Input: part model. Units: mm. Frame: model coordinates. Face numbers are marked on the shaded views. A direction names the side the tool comes from. Coordinates: 2 decimals unless noted, no trailing zeros. Order: outer loops, then holes, each group sorted by start corner. A loop starts at its lowest first (then second) coordinate and runs counter-clockwise, first axis right, second up. Notation, with made-up numbers: M -15.5,45 L 17.5,45 A25 ccw 17.5,63 Z; hole C 28.25,29 d7. An arc over 180 degrees is marked long. One line per item, written item: value.
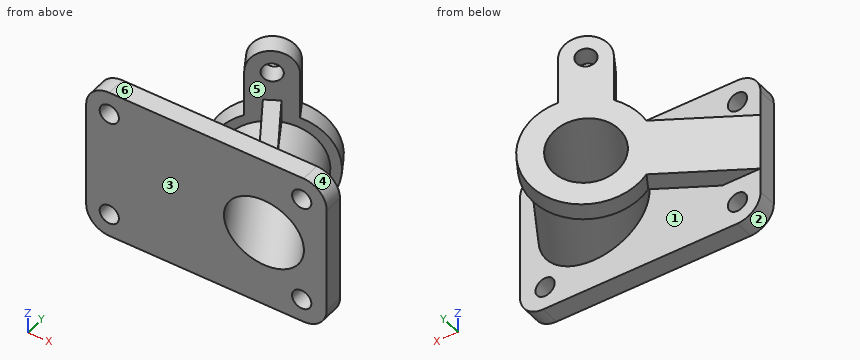
```python
from build123d import *

# Parameters (mm, degrees)
SKETCH_1_R          = 5
EXTRUDE_1_DEPTH     = 10
SKETCH_3_R          = 5
SKETCH_3_R_2        = 18
EXTRUDE_3_DEPTH     = 10
EXTRUDE_4_REACH     = 73.16
SKETCH_4_R          = 25
SKETCH_5_R          = 18
CUT_EXTRUDE_1_DEPTH = 72.160254038
EXTRUDE_6_DEPTH     = 4


with BuildPart() as part:
    # 草图1 → 凸台-拉伸1 (new body)
    with BuildSketch(Plane(origin=(0, 0, 0), x_dir=(1, 0, 0), z_dir=(0, 1, 0))):
        with BuildLine():
            Line((-69.708508874, 31.297621281), (31.291491126, 31.297621281))
            ThreePointArc((31.291491126, 31.297621281), (39.7767725, 27.782902656), (43.291491126, 19.297621281))
            Line((43.291491126, 19.297621281), (43.291491126, -36.702378719))
            ThreePointArc((43.291491126, -36.702378719), (39.7767725, -45.187660093), (31.291491126, -48.702378719))
            Line((31.291491126, -48.702378719), (-69.708508874, -48.702378719))
            ThreePointArc((-69.708508874, -48.702378719), (-78.193790248, -45.187660093), (-81.708508874, -36.702378719))
            Line((-81.708508874, -36.702378719), (-81.708508874, 19.297621281))
            ThreePointArc((-81.708508874, 19.297621281), (-78.193790248, 27.782902656), (-69.708508874, 31.297621281))
        make_face()
        with Locations((-69.708508874, -36.702378719)):
            Circle(SKETCH_1_R, mode=Mode.SUBTRACT)
        with Locations((30.291491126, -36.702378719)):
            Circle(SKETCH_1_R, mode=Mode.SUBTRACT)
        with Locations((30.291491126, 19.297621281)):
            Circle(SKETCH_1_R, mode=Mode.SUBTRACT)
        with Locations((-69.708508874, 19.297621281)):
            Circle(SKETCH_1_R, mode=Mode.SUBTRACT)
    extrude(amount=EXTRUDE_1_DEPTH)

    # 草图3 → 凸台-拉伸3 (add)
    with BuildSketch(Plane(origin=(-24.757254237, 42.880822195, 0), x_dir=(0, 0, 1), z_dir=(-0.5, 0.866025404, 0))):
        with BuildLine():
            Line((-6.297621281, -65.76164439), (-6.297621281, -16.742406504))
            ThreePointArc((-6.297621281, -16.742406504), (-11.289336226, 31.606443002), (36.197832888, 21.23835561))
            Line((36.197832888, 21.23835561), (60.702378719, 21.23835561))
            ThreePointArc((60.702378719, 21.23835561), (72.702378719, 9.23835561), (60.702378719, -2.76164439))
            Line((60.702378719, -2.76164439), (36.197832888, -2.76164439))
            ThreePointArc((36.197832888, -2.76164439), (31.070466111, -10.753359335), (23.702378719, -16.742406504))
            Line((23.702378719, -16.742406504), (23.702378719, -65.76164439))
            Line((23.702378719, -65.76164439), (-6.297621281, -65.76164439))
        make_face()
        with Locations((60.702378719, 9.23835561)):
            Circle(SKETCH_3_R, mode=Mode.SUBTRACT)
        with Locations((8.702378719, 9.23835561)):
            Circle(SKETCH_3_R_2, mode=Mode.SUBTRACT)
    extrude(amount=-EXTRUDE_3_DEPTH)

    # 草图4 → 凸台-拉伸4 (add, up to next)
    with BuildSketch(Plane(origin=(-24.757254237, 42.880822195, 0), x_dir=(0, 0, 1), z_dir=(-0.5, 0.866025404, 0)), mode=Mode.PRIVATE) as extrude_4_sk1:
        with Locations((8.702378719, 9.23835561)):
            Circle(SKETCH_4_R)
    extrude_4_tool1 = extrude(extrude_4_sk1.sketch, amount=-EXTRUDE_4_REACH, mode=Mode.PRIVATE) - part.part
    add(extrude_4_tool1.solids().sort_by_distance((-16.756604, 47.5, 8.702379))[0])

    # 草图5 → 切除-拉伸1 (cut, through all)
    with BuildSketch(Plane(origin=(-24.757254237, 42.880822195, 0), x_dir=(0.866025404, 0.5, 0), z_dir=(-0.5, 0.866025404, 0))):
        with Locations((9.23835561, -8.702378719)):
            Circle(SKETCH_5_R)
    extrude(amount=-CUT_EXTRUDE_1_DEPTH, mode=Mode.SUBTRACT)

    # 草图7 → 凸台-拉伸6 (add, symmetric)
    with BuildSketch(Plane(origin=(8.000650647, 4.619177805, 0), x_dir=(0, 0, 1), z_dir=(-0.866025404, -0.5, 0))):
        Polygon((45.297720901, 39.514508475), (30.011923646, 39.514508475), (30.472342637, 13.83620008), align=None)
    extrude(amount=EXTRUDE_6_DEPTH, both=True)


solid = part.part
```
(1) Access query for the marked faces 4, 5 and 6. Directions: +Z, -Z, +X, -X, +Y, -Y. A direction counts if a zero-diameter tool reaches every point of the face in a straight line with its end or side. Return the directions, or none.
Data:
face 4: +Z, +X, +Y, -Y
face 5: none
face 6: +Z, +X, -X, -Y
(2) First-contact query: pin 1 (8 mm diameter, centred on y = 16.5, z = -11, fed in from +X) (3 decimals); pin 2 (10 mm diameter, centred on x = 7.5, y = 56, fed in from +Z); pin 3 (1 mm diameter, centred on x = 27.5, z = 16, fed in from -Y); pin 4 (13 mm diameter, centred on x = 30.29, z = 36.7, fed in from -Y). Flat tips, straight axial feed; report the tip coordinate or a pass-through.
Data:
pin 1: stops at x = 24.245
pin 2: stops at z = 30.83
pin 3: stops at y = 2.78
pin 4: stops at y = 0
(3) Draft query along X for the marked faces 1, 2 and 3. Return one class per face: released by +X, released by -X, zero draft, split by the parting line, or undercut.
Data:
face 1: undercut
face 2: released by -X
face 3: zero draft
(4) Cut plane A-A on z = 16. Output: boundary loops of the cut face in (x, y).
Data:
outline: M -81.71,0 L -8.33,0 L -31.01,39.27 L -81.71,10 Z; M -2.51,55.73 L 29.67,0 L 43.29,0 L 43.29,10 L 32.5,10 L 8.95,50.8 L 13.44,53.39 L 8.44,62.05 Z; hole M -61.71,10 L -22.72,10 L -32.46,26.88 Z
(5) Cut plane C-C on x = -45. Output: boundary loops of the cut face in (y, z).
Data:
outline: M 0,-31.3 L 10,-31.3 L 10,48.7 L 0,48.7 Z; M 19.65,-6.3 L 31.19,-6.3 L 31.19,23.7 L 19.65,23.7 Z
(6) Cut plane B-B on x = -67. Output: boundary loops of the cut face in (y, z).
Data:
outline: M 0,-31.3 L 10,-31.3 L 10,-23.5 L 0,-23.5 Z; M 0,-15.09 L 10,-15.09 L 10,-6.3 L 18.49,-6.3 L 18.49,23.7 L 10,23.7 L 10,32.5 L 0,32.5 Z; M 0,40.91 L 10,40.91 L 10,48.7 L 0,48.7 Z
(7) Ray query, line 1 (Z direction, x = -13, y = 46); line 2 (Z direction, x = 8, y = 4); line 3 (X direction, y = 27, z = 0). Return the intervals inside material, ascending. Write a range as from..to.
Data:
line 1: z = -21.19..-9.12, 26.53..56.37, 65.03..72.44
line 2: z = -31.3..-9.29, 26.7..48.7
line 3: x = -52.26..-32.26, -31.98..-23.12, 13.27..22.14
(8) Cut plane D-D on z = 1.5. Output: boundary loops of the cut face in (x, y), plus the area to 3 significant figures.
Data:
outline: M -81.71,0 L -8.38,0 L -31.04,39.25 L -81.71,10 Z; M -2.47,55.75 L 29.72,0 L 43.29,0 L 43.29,10 L 32.54,10 L 8.98,50.81 L 13.46,53.4 L 8.46,62.06 Z; hole M -61.71,10 L -22.75,10 L -32.49,26.87 Z
area: 1,990 mm2
